The model under review builds one solid part; all positions refer to its coordinate system, in mm. A direction names the side the tool comes from. Round coordinates to 2 decimals unless told otherwise and drop trailing zeros. Order: outer loops, then holes, each group sorted by start corner. A loop starts at its lowest first (then second) coordinate and runs counter-clockwise, first axis right, second up.
```python
from build123d import *

# Parameters (mm, degrees)
ESQUISSE1_W                             = 70
ESQUISSE1_H                             = 30
T_LE_DE_BASE_PLI_E1_DEPTH               = 1
T_LE_PLI_E_SUR_AR_TE1_STRIP_W           = 5.4732
T_LE_PLI_E_SUR_AR_TE1_STRIP_H           = 1
T_LE_PLI_E_SUR_AR_TE1_STRIP_CUT_DEPTH   = 30
T_LE_PLI_E_SUR_AR_TE1_STRIP_2_W         = 5.4732
T_LE_PLI_E_SUR_AR_TE1_STRIP_2_H         = 1
T_LE_PLI_E_SUR_AR_TE1_STRIP_CUT_2_DEPTH = 30
T_LE_PLI_E_SUR_AR_TE1_DEPTH             = 30
T_LE_PLI_E_SUR_AR_TE1_BEND_DEPTH        = 30
T_LE_PLI_E_SUR_AR_TE2_STRIP_W           = 5.4732
T_LE_PLI_E_SUR_AR_TE2_STRIP_H           = 1
T_LE_PLI_E_SUR_AR_TE2_STRIP_CUT_DEPTH   = 30
T_LE_PLI_E_SUR_AR_TE2_STRIP_2_W         = 5.4732
T_LE_PLI_E_SUR_AR_TE2_STRIP_2_H         = 1
T_LE_PLI_E_SUR_AR_TE2_STRIP_CUT_2_DEPTH = 30
T_LE_PLI_E_SUR_AR_TE2_DEPTH             = 30
T_LE_PLI_E_SUR_AR_TE2_BEND_DEPTH        = 30
ENL_V_MAT_EXTRU_1_REACH                 = 45.486
ESQUISSE12_R                            = 1.7
ENL_V_MAT_EXTRU_3_REACH                 = 45.012
ESQUISSE27_R                            = 2.25


# Sheet-metal steps are written as plain solids
with BuildPart() as part:
    # Esquisse1 → Tôle de base pliée1 (new body)
    with BuildSketch(Plane(origin=(0, 0, 0), x_dir=(1, 0, 0), z_dir=(0, 1, 0))):
        Rectangle(ESQUISSE1_W, ESQUISSE1_H)
    extrude(amount=T_LE_DE_BASE_PLI_E1_DEPTH)

    # Tôle pliée sur arête1 strip (across the edge) → Tôle pliée sur arête1 strip cut (cut)
    with BuildSketch(Plane(origin=(-35, 1, -15), x_dir=(1, 0, 0), z_dir=(0, 0, 1))):
        with Locations((-1, -0.5)):
            Rectangle(T_LE_PLI_E_SUR_AR_TE1_STRIP_W, T_LE_PLI_E_SUR_AR_TE1_STRIP_H)
    extrude(amount=T_LE_PLI_E_SUR_AR_TE1_STRIP_CUT_DEPTH, mode=Mode.SUBTRACT)

    # Tôle pliée sur arête1 strip 2 (across the edge) → Tôle pliée sur arête1 strip cut 2 (cut)
    with BuildSketch(Plane(origin=(35, 1, 15), x_dir=(-1, 0, 0), z_dir=(0, 0, -1))):
        with Locations((-1, -0.5)):
            Rectangle(T_LE_PLI_E_SUR_AR_TE1_STRIP_2_W, T_LE_PLI_E_SUR_AR_TE1_STRIP_2_H)
    extrude(amount=T_LE_PLI_E_SUR_AR_TE1_STRIP_CUT_2_DEPTH, mode=Mode.SUBTRACT)

    # Tôle pliée sur arête1 section (across the edge) → Tôle pliée sur arête1 (add)
    with BuildSketch(Plane(origin=(-35, 1, -15), x_dir=(1, 0, 0), z_dir=(0, 0, 1))):
        with BuildLine():
            Line((0, 0.7366), (0, 20))
            Line((0, 20), (1, 20))
            Line((1, 20), (1, 0.7366))
            ThreePointArc((1, 0.7366), (1.215745145, 0.215745145), (1.7366, 0))
            Line((1.7366, 0), (1.7366, -1))
            ThreePointArc((1.7366, -1), (0.508638364, -0.491361636), (0, 0.7366))
        make_face()
    extrude(amount=T_LE_PLI_E_SUR_AR_TE1_DEPTH)

    # Tôle pliée sur arête1 section 2 (across the edge) → Tôle pliée sur arête1 bend (add)
    with BuildSketch(Plane(origin=(35, 1, 15), x_dir=(-1, 0, 0), z_dir=(0, 0, -1))):
        with BuildLine():
            Line((0, 0.7366), (0, 20))
            Line((0, 20), (1, 20))
            Line((1, 20), (1, 0.7366))
            ThreePointArc((1, 0.7366), (1.215745145, 0.215745145), (1.7366, 0))
            Line((1.7366, 0), (1.7366, -1))
            ThreePointArc((1.7366, -1), (0.508638364, -0.491361636), (0, 0.7366))
        make_face()
    extrude(amount=T_LE_PLI_E_SUR_AR_TE1_BEND_DEPTH)

    # Tôle pliée sur arête2 strip (across the edge) → Tôle pliée sur arête2 strip cut (cut)
    with BuildSketch(Plane(origin=(-34, 21, -15), x_dir=(0, -1, 0), z_dir=(0, 0, 1))):
        with Locations((-1, -0.5)):
            Rectangle(T_LE_PLI_E_SUR_AR_TE2_STRIP_W, T_LE_PLI_E_SUR_AR_TE2_STRIP_H)
    extrude(amount=T_LE_PLI_E_SUR_AR_TE2_STRIP_CUT_DEPTH, mode=Mode.SUBTRACT)

    # Tôle pliée sur arête2 strip 2 (across the edge) → Tôle pliée sur arête2 strip cut 2 (cut)
    with BuildSketch(Plane(origin=(34, 21, 15), x_dir=(0, -1, 0), z_dir=(0, 0, -1))):
        with Locations((-1, -0.5)):
            Rectangle(T_LE_PLI_E_SUR_AR_TE2_STRIP_2_W, T_LE_PLI_E_SUR_AR_TE2_STRIP_2_H)
    extrude(amount=T_LE_PLI_E_SUR_AR_TE2_STRIP_CUT_2_DEPTH, mode=Mode.SUBTRACT)

    # Tôle pliée sur arête2 section (across the edge) → Tôle pliée sur arête2 (add)
    with BuildSketch(Plane(origin=(-34, 21, -15), x_dir=(0, -1, 0), z_dir=(0, 0, 1))):
        with BuildLine():
            Line((0, 0.7366), (0, 8))
            Line((0, 8), (1, 8))
            Line((1, 8), (1, 0.7366))
            ThreePointArc((1, 0.7366), (1.215745145, 0.215745145), (1.7366, 0))
            Line((1.7366, 0), (1.7366, -1))
            ThreePointArc((1.7366, -1), (0.508638364, -0.491361636), (0, 0.7366))
        make_face()
    extrude(amount=T_LE_PLI_E_SUR_AR_TE2_DEPTH)

    # Tôle pliée sur arête2 section 2 (across the edge) → Tôle pliée sur arête2 bend (add)
    with BuildSketch(Plane(origin=(34, 21, 15), x_dir=(0, -1, 0), z_dir=(0, 0, -1))):
        with BuildLine():
            Line((0, 0.7366), (0, 8))
            Line((0, 8), (1, 8))
            Line((1, 8), (1, 0.7366))
            ThreePointArc((1, 0.7366), (1.215745145, 0.215745145), (1.7366, 0))
            Line((1.7366, 0), (1.7366, -1))
            ThreePointArc((1.7366, -1), (0.508638364, -0.491361636), (0, 0.7366))
        make_face()
    extrude(amount=T_LE_PLI_E_SUR_AR_TE2_BEND_DEPTH)

    # Esquisse12 → Enlèv. mat.-Extru.1 (cut, up to next)
    with BuildSketch(Plane(origin=(0, 21, 0), x_dir=(1, 0, 0), z_dir=(0, 1, 0)), mode=Mode.PRIVATE) as enl_v_mat_extru_1_sk1:
        with Locations(Location((-30, 0, 0), (0, 0, 180))):
            Circle(ESQUISSE12_R)
    enl_v_mat_extru_1_tool1 = extrude(enl_v_mat_extru_1_sk1.sketch, amount=-ENL_V_MAT_EXTRU_1_REACH, mode=Mode.PRIVATE) & part.part
    # Esquisse12 → Enlèv. mat.-Extru.1 (cut, up to next)
    with BuildSketch(Plane(origin=(0, 21, 0), x_dir=(1, 0, 0), z_dir=(0, 1, 0)), mode=Mode.PRIVATE) as enl_v_mat_extru_1_sk2:
        with Locations(Location((30, 10, 0), (0, 0, 180))):
            Circle(ESQUISSE12_R)
    enl_v_mat_extru_1_tool2 = extrude(enl_v_mat_extru_1_sk2.sketch, amount=-ENL_V_MAT_EXTRU_1_REACH, mode=Mode.PRIVATE) & part.part
    # Esquisse12 → Enlèv. mat.-Extru.1 (cut, up to next)
    with BuildSketch(Plane(origin=(0, 21, 0), x_dir=(1, 0, 0), z_dir=(0, 1, 0)), mode=Mode.PRIVATE) as enl_v_mat_extru_1_sk3:
        with Locations(Location((30, -10, 0), (0, 0, 180))):
            Circle(ESQUISSE12_R)
    enl_v_mat_extru_1_tool3 = extrude(enl_v_mat_extru_1_sk3.sketch, amount=-ENL_V_MAT_EXTRU_1_REACH, mode=Mode.PRIVATE) & part.part
    add(enl_v_mat_extru_1_tool1.solids().sort_by_distance((-30, 21, 0))[0], mode=Mode.SUBTRACT)
    add(enl_v_mat_extru_1_tool2.solids().sort_by_distance((30, 21, -10))[0], mode=Mode.SUBTRACT)
    add(enl_v_mat_extru_1_tool3.solids().sort_by_distance((30, 21, 10))[0], mode=Mode.SUBTRACT)

    # Esquisse27 → Enlèv. mat.-Extru.3 (cut, up to next)
    with BuildSketch(Plane(origin=(0, 1, 0), x_dir=(1, 0, 0), z_dir=(0, 1, 0)), mode=Mode.PRIVATE) as enl_v_mat_extru_3_sk1:
        with Locations(Location((-20, 0, 0), (0, 0, 270))):
            Circle(ESQUISSE27_R)
    enl_v_mat_extru_3_tool1 = extrude(enl_v_mat_extru_3_sk1.sketch, amount=-ENL_V_MAT_EXTRU_3_REACH, mode=Mode.PRIVATE) & part.part
    # Esquisse27 → Enlèv. mat.-Extru.3 (cut, up to next)
    with BuildSketch(Plane(origin=(0, 1, 0), x_dir=(1, 0, 0), z_dir=(0, 1, 0)), mode=Mode.PRIVATE) as enl_v_mat_extru_3_sk2:
        with Locations(Location((20, 0, 0), (0, 0, 90))):
            Circle(ESQUISSE27_R)
    enl_v_mat_extru_3_tool2 = extrude(enl_v_mat_extru_3_sk2.sketch, amount=-ENL_V_MAT_EXTRU_3_REACH, mode=Mode.PRIVATE) & part.part
    add(enl_v_mat_extru_3_tool1.solids().sort_by_distance((-20, 1, 0))[0], mode=Mode.SUBTRACT)
    add(enl_v_mat_extru_3_tool2.solids().sort_by_distance((20, 1, 0))[0], mode=Mode.SUBTRACT)


solid = part.part
```
(1) Consider section B-B (z = 10). Write out the cut boundary in (x, y).
Data:
outline: (-35, 1.74) arc R1.74 ccw to (-33.26, 0) - (33.26, 0) arc R1.74 ccw to (35, 1.74) - (35, 19.26) arc R1.74 ccw to (33.26, 21) - (31.7, 21) - (31.7, 20) - (33.26, 20) arc R0.74 cw to (34, 19.26) - (34, 1.74) arc R0.74 cw to (33.26, 1) - (-33.26, 1) arc R0.74 cw to (-34, 1.74) - (-34, 19.26) arc R0.74 cw to (-33.26, 20) - (-26, 20) - (-26, 21) - (-33.26, 21) arc R1.74 ccw to (-35, 19.26) - close; (26, 20) - (28.3, 20) - (28.3, 21) - (26, 21) - close
(2) For faces 5 (the cylindrical face through (-22.196, 0.507, -0.488)), 6 (the flat face through (-34, 11, 0)), 7 (the cylindrical face through (-31.57, 20.51, -0.65)), list the 3-axis set-ups (+Z, -Z, +X, -X, +Y, -Y) from which the entire face can be reached by the end or side of a thin tool; tool diameter is ignored.
Data:
face 5: +Y, -Y
face 6: +Z, -Z
face 7: +Y
(3) Consider section D-D (y = 5). Write out the cut boundary in (x, z), and give its area (3 significant figures).
Data:
outline: (-35, -15) - (-34, -15) - (-34, 15) - (-35, 15) - close; (34, -15) - (35, -15) - (35, 15) - (34, 15) - close
area: 60.0 mm2
(4) Insertion check: pin 1 (1 mm diameter, centred on x = -2, z = 1, fed in from -Y); pin 2 (8 mm diameter, centred on x = 20, z = 11.5, fed in from +Y); pin 3 (10 mm diameter, centred on x = 23.5, y = 14.5, fed in from +Z); pin 4 (0.5 mm diameter, centred on y = 20.5, z = -1.5, fed in from +X). Each pin has a flat end and moves straight along its axis. Give the tip position at first contact, or say it passes through.
Data:
pin 1: stops at y = 0
pin 2: stops at y = 1
pin 3: passes through
pin 4: stops at x = 34.69
(5) Consider section C-C (z = 0). State how many separate pieces and enclosed holes the cut face has, and give its area (3 significant figures).
Data:
separate pieces: 4
enclosed holes: 0
area: 111 mm2
(6) Draft analysis for pull direction X (two halves, no side actions). For faces 1 (the flat face through (30, 20, 0)), 2 (the flat face through (0, 1, 0)), 3 (the flat face through (30, 21, 0)), 4 (the flat face through (35, 10, 0)), state which applies: pulls with the +X half, pulls with the -X half, needs draft (parallel to the pull), parting line crosses it, or undercut.
Data:
face 1: undercut
face 2: undercut
face 3: needs draft
face 4: pulls with the +X half
(7) Consider section A-A (x = 30). Write out the cut boundary in (y, z).
Data:
outline: (0, -15) - (1, -15) - (1, 15) - (0, 15) - close; (20, -15) - (21, -15) - (21, -11.7) - (20, -11.7) - close; (20, -8.3) - (21, -8.3) - (21, 8.3) - (20, 8.3) - close; (20, 11.7) - (21, 11.7) - (21, 15) - (20, 15) - close
(8) To check wall thickness, follow probe 1 along Z at (x, y) = (30, 20.6); probe 2 along X at (y, z) = (7.5, 13); probe 3 along X at (y, z) = (0.7, 0). State the ranges of each line that lie inside material, in increasing order.
Data:
probe 1: z = -15 to -11.7, -8.3 to 8.3, 11.7 to 15
probe 2: x = -35 to -34, 34 to 35
probe 3: x = -34.66 to -22.25, -17.75 to 17.75, 22.25 to 34.66
